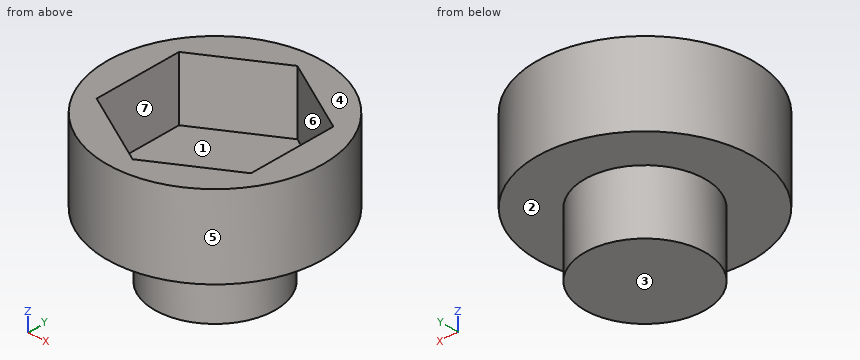
```python
from build123d import *

# Parameters (mm, degrees)
SKETCH_R     = 17
PAD_DEPTH    = 3
SKETCH001_R  = 17
PAD001_DEPTH = 10
SKETCH002_R  = 9.49
PAD002_DEPTH = 10


with BuildPart() as part:
    # Sketch → Pad (new body)
    with BuildSketch(Plane.XY):
        Circle(SKETCH_R)
    extrude(amount=PAD_DEPTH)

    # Sketch001 (on Face3 of Pad) → Pad001 (join)
    with BuildSketch(Plane.XY.offset(3)):
        Circle(SKETCH001_R)
        Polygon((0, 14.1), (-12.210958, 7.05), (-12.210958, -7.05), (0, -14.1), (12.210958, -7.05), (12.210958, 7.05), align=None, mode=Mode.SUBTRACT)
    extrude(amount=PAD001_DEPTH)

    # Sketch002 (on Face2 of Pad001) → Pad002 (join)
    with BuildSketch(Plane(origin=(0, 0, 0), x_dir=(1, 0, 0), z_dir=(0, 0, -1))):
        Circle(SKETCH002_R)
    extrude(amount=PAD002_DEPTH)


solid = part.part
```
The listing builds one solid part. Answer for the finished solid, in the listing's coordinates (mm). Face numbers are marked on the shaded views. A direction names the side the tool comes from. Round coordinates to 2 decimals unless told otherwise and drop trailing zeros. Write each loop counter-clockwise with the first axis right and the second up, starting at its lowest first coordinate (ties: lowest second). Pieces come first, ordered by that corner, then holes. Notation, with made-up numbers: (-25.75, -7.5) -> (26.25, -7.5) arc R28 cw to (26.25, 12.5) -> close; hole circle Ø10 at (29.25, 6.25). An arc over 180 degrees is marked (long way). Write item = value, one per line.
1) Straight lines are drawn through the part: line 1 along X through (y, z) = (0.5, 11); line 2 along Z through (x, y) = (-7.5, 10.5); line 3 along Z through (x, y) = (-2, -4). For each, find the intervals that lie inside material, in ascending order. Write a range as [from, to].
Check values:
line_1 = [-16.99, -12.21], [12.21, 16.99]
line_2 = [0, 13]
line_3 = [-10, 3]
2) Given pin 1 (1 mm diameter, centred on y = -2, z = 2, fed in from -X); pin 2 (7.5 mm diameter, centred on x = 5.5, y = -5, fed in from +Z); pin 3 (5 mm diameter, centred on y = -13, z = 10.5, fed in from +X), each flat-ended and moving along its own axis, determine where each tip first touches the part or whether it passes through.
Check values:
pin_1 = -16.93
pin_2 = 3
pin_3 = 13.37
3) Section C-C on y = -3 is taken. Write down the section's boundary in (x, z).
Check values:
outline = (-16.73, 0) -> (-9, 0) -> (-9, -10) -> (9, -10) -> (9, 0) -> (16.73, 0) -> (16.73, 13) -> (12.21, 13) -> (12.21, 3) -> (-12.21, 3) -> (-12.21, 13) -> (-16.73, 13) -> close
4) Section B-B on x = 11.5 is taken. Write down the section's boundary in (y, z).
Check values:
outline = (-12.52, 0) -> (12.52, 0) -> (12.52, 13) -> (7.46, 13) -> (7.46, 3) -> (-7.46, 3) -> (-7.46, 13) -> (-12.52, 13) -> close
5) For a pull along X with two mould halves and no side action, classify the marked faces 4, 5, 6 and 7 as released by +X, released by -X, zero draft, split by the parting line, or undercut.
Check values:
face_4 = zero draft
face_5 = split by the parting line
face_6 = undercut
face_7 = undercut
6) Section A-A on z = 6.5 is taken. Write down the section's boundary in (x, y), plus the area to 3 significant figures.
Check values:
outline = circle Ø34 at (0, 0); hole (-12.21, -7.05) -> (0, -14.1) -> (12.21, -7.05) -> (12.21, 7.05) -> (0, 14.1) -> (-12.21, 7.05) -> close
area = 391 mm²
7) Section D-D on z = -8.5 is taken. Write down the section's boundary in (x, y).
Check values:
outline = circle Ø18.98 at (0, 0)
8) Which of the six approach directions +Z, -Z, +X, -X, +Y, -Y give full straight-line access (tool end or side, diameter ignored) to the marked faces 1, 2 and 3?
Check values:
face_1 = +Z
face_2 = -Z
face_3 = -Z, +X, -X, +Y, -Y
